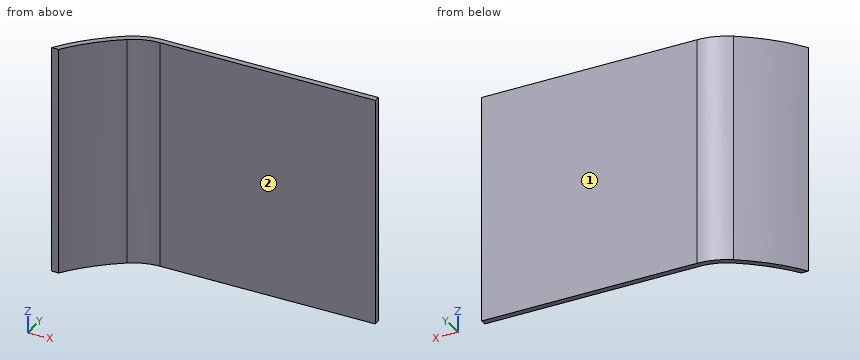
```python
from build123d import *

# Parameters (mm, degrees)
F0_W     = 101.6
F0_H     = 101.6
F1_DEPTH = 12.7
F3_DEPTH = 101.6
F4_R     = 25.4
F5_T     = -2.54


# Not quite as in the source:
# - a feature of the source that left no trace in its solid (it failed there, or was rolled back) is left out


with BuildPart() as f1:
    # F0 (on Front) → F1 (new body, symmetric)
    with BuildSketch(Plane.XZ):
        with Locations((1.211412394, -8.554763478)):
            Rectangle(F0_W, F0_H)
    extrude(amount=F1_DEPTH, both=True)

    # F2 (on face) → F3 (join)
    with BuildSketch(Plane.XY.offset(42.245236522)):
        with BuildLine():
            Line((-49.588587606, -12.7), (-49.588587606, 12.7))
            add(Edge.make_bspline(
                [(-49.588587606, 12.7), (-67.7978310293, 3.2621913661), (-78.5642321364, -12.7)],
                knots=[1.1900846756, 1.1900846756, 1.1900846756, 2.1282604502, 2.1282604502, 2.1282604502], degree=2, weights=[1, 0.8919810006, 1]))
            Line((-78.5642321364, -12.7), (-49.588587606, -12.7))
        make_face()
    extrude(amount=-F3_DEPTH)

    # F4
    f4_edges = [f1.edges().sort_by_distance(p)[0] for p in [
        (-49.588588, 12.7, -8.554763),
    ]]
    fillet(f4_edges, radius=F4_R)

    # F5
    f5_openings = [f1.faces().sort_by_distance(p)[0] for p in [
        (-7.437576, -0.524073, 42.245237),
        (-13.27641, -12.7, -8.554763),
        (52.011412, 0, -8.554763),
        (-7.437576, -0.524073, -59.354763),
    ]]
    offset(amount=F5_T, openings=f5_openings)


solid = f1.part
```
Read the model definition and answer for the solid it produces. Units are mm, in the model's axes. Face numbers are marked on the shaded views. A direction names the side the tool comes from. Coordinates: 2 decimals unless noted, no trailing zeros. Write each loop counter-clockwise with the first axis right and the second up, starting at its lowest first coordinate (ties: lowest second). Pieces come first, ordered by that corner, then holes. Notation, with made-up numbers: (62, 0.25) - (96, 0.25) arc R24 ccw to (96, 12.25) - close; hole circle Ø10 at (-1, -38.5). An arc over 180 degrees is marked (long way). Answer as a JSON object with one key per item and string values. Group by question number.
1. A cutting plane is placed at A-A (x = 7). Determine the outline of the cut face in (y, z).
2. Each of these flat-tipped pins is pushed along its axis until it touches: P1, Ø8, axis at y = -7.5, z = -33.5, coming from the +X side; P2, Ø5, axis at y = -3, z = -24.5, coming from the -X side; P3, Ø6, axis at x = 5, z = 27, coming from the -Y side; P4, Ø2, axis at x = -48, y = 9.5, coming from the -Z side. Where does it stop, or does it pass through?
3. Which of the six approach directions +Z, -Z, +X, -X, +Y, -Y give full straight-line access (tool end or side, diameter ignored) to the marked faces 1 and 2?
4. Consider L1, parallel to Y at x = 4, z = 18; L2, parallel to X at y = -9.5, z = -52; L3, parallel to X at y = 5, z = -19. Determine where each line is inside the solid, lowest interval first. Write a range as [from, to].
Worked out:
{
 "1": {"outline": "(10.16, -59.35) - (12.7, -59.35) - (12.7, 42.25) - (10.16, 42.25) - close"},
 "2": {"P1": "stops at x = -67.53", "P2": "stops at x = -72.94", "P3": "stops at y = 10.16", "P4": "stops at z = -59.35"},
 "3": {"face 1": "+Z, -Z, +X, -X, +Y", "face 2": "+Z, -Z, +X, -Y"},
 "4": {"L1": "y = [10.16, 12.7]", "L2": "x = [-76.26, -73.02]", "L3": "x = [-61.62, -57.34]"}
}
